Source: CAD feature listing. Evaluate the final solid. Frame: model axes, mm. A direction names the side the tool comes from. Round coordinates to 2 decimals unless told otherwise and drop trailing zeros. Return JSON: item names as keys, results as strings. Group by question number.
```python
from build123d import *
from build123d.topology import SkipClean

# Parameters (mm, degrees)
SKETCH1_R           = 8.984375
SKETCH1_R_2         = 1.984375
SKETCH1_R_3         = 0.75
BOSS_EXTRUDE1_DEPTH = 2
SKETCH6_W           = 17.96875
SKETCH6_H           = 8
CUT_EXTRUDE1_DEPTH  = 16.014592511
BOSS_EXTRUDE3_START = -2
SKETCH7_R           = 1.65
BOSS_EXTRUDE3_DEPTH = 2
SKETCH8_R           = 1.1
BOSS_EXTRUDE4_DEPTH = 1


with BuildPart() as part:
    # Sketch1 → Boss-Extrude1 (new body)
    with BuildSketch(Plane(origin=(0, 0, 0), x_dir=(1, 0, 0), z_dir=(0, 1, 0))):
        with Locations(Location((0, 0, 0), (0, 0, 270))):
            Circle(SKETCH1_R)
        with Locations(Location((0, 0, 0), (0, 0, 270))):
            Circle(SKETCH1_R_2, mode=Mode.SUBTRACT)
        with Locations(Location((0, 7, 0), (0, 0, 270))):
            Circle(SKETCH1_R_3, mode=Mode.SUBTRACT)
        with Locations(Location((5.472820377, 4.364428613, 0), (0, 0, 270))):
            Circle(SKETCH1_R_3, mode=Mode.SUBTRACT)
        with Locations(Location((6.824495385, -1.557646538, 0), (0, 0, 270))):
            Circle(SKETCH1_R_3, mode=Mode.SUBTRACT)
        with Locations(Location((3.037186174, -6.306782075, 0), (0, 0, 270))):
            Circle(SKETCH1_R_3, mode=Mode.SUBTRACT)
        with Locations(Location((-3.037186174, -6.306782075, 0), (0, 0, 270))):
            Circle(SKETCH1_R_3, mode=Mode.SUBTRACT)
        with Locations(Location((-6.824495385, -1.557646538, 0), (0, 0, 270))):
            Circle(SKETCH1_R_3, mode=Mode.SUBTRACT)
        with Locations(Location((-5.472820377, 4.364428613, 0), (0, 0, 270))):
            Circle(SKETCH1_R_3, mode=Mode.SUBTRACT)
    extrude(amount=BOSS_EXTRUDE1_DEPTH)

    # Sweep1: sweep along a path in Sketch3
    with SkipClean():  # the faces are left unmerged after this step: merging them gives an invalid solid
        with BuildLine(Plane(origin=(0, 0, 0), x_dir=(0, 0, -1), z_dir=(1, 0, 0))) as sweep1_path:
            Line((0, 2), (0, 8))
        # Sketch2 → Sweep1 (sweep)
        with BuildSketch(Plane(origin=(0, 2, 0), x_dir=(1, 0, 0), z_dir=(0, 1, 0))):
            with BuildLine():
                Line((-0.5, 6.229967897), (-0.5, 1.920350005))
                ThreePointArc((-0.5, 1.920350005), (-0.860988045, 1.787860097), (-1.18964519, 1.588234385))
                Line((-1.18964519, 1.588234385), (-4.559040136, 4.275237191))
                ThreePointArc((-4.559040136, 4.275237191), (-2.711773369, 5.631055424), (-0.5, 6.229967897))
            make_face()
            with BuildLine():
                Line((0.5, 6.229967897), (0.5, 1.920350005))
                ThreePointArc((0.5, 1.920350005), (0.860988045, 1.787860097), (1.18964519, 1.588234385))
                Line((1.18964519, 1.588234385), (4.559040136, 4.275237191))
                ThreePointArc((4.559040136, 4.275237191), (2.711773369, 5.631055424), (0.5, 6.229967897))
            make_face()
            with BuildLine():
                Line((5.182529938, 3.493405709), (1.813134992, 0.806402903))
                ThreePointArc((1.813134992, 0.806402903), (1.934622576, 0.441564978), (1.983463288, 0.06014588))
                Line((1.983463288, 0.06014588), (6.185030062, -0.898834319))
                ThreePointArc((6.185030062, -0.898834319), (6.093299451, 1.390755837), (5.182529938, 3.493405709))
            make_face()
            with BuildLine():
                Line((5.962509128, -1.873762231), (1.760942354, -0.914782033))
                ThreePointArc((1.760942354, -0.914782033), (1.551446848, -1.237237576), (1.283693074, -1.5132337))
                Line((1.283693074, -1.5132337), (3.1535662, -5.396065254))
                ThreePointArc((3.1535662, -5.396065254), (4.886446765, -3.896811262), (5.962509128, -1.873762231))
            make_face()
            with BuildLine():
                Line((2.252597332, -5.829948993), (0.382724207, -1.947117439))
                ThreePointArc((0.382724207, -1.947117439), (0, -1.984375), (-0.382724207, -1.947117439))
                Line((-0.382724207, -1.947117439), (-2.252597332, -5.829948993))
                ThreePointArc((-2.252597332, -5.829948993), (0, -6.25), (2.252597332, -5.829948993))
            make_face()
            with BuildLine():
                Line((-3.1535662, -5.396065254), (-1.283693074, -1.5132337))
                ThreePointArc((-1.283693074, -1.5132337), (-1.551446848, -1.237237576), (-1.760942354, -0.914782033))
                Line((-1.760942354, -0.914782033), (-5.962509128, -1.873762231))
                ThreePointArc((-5.962509128, -1.873762231), (-4.886446765, -3.896811262), (-3.1535662, -5.396065254))
            make_face()
            with BuildLine():
                Line((-6.185030062, -0.898834319), (-1.983463288, 0.06014588))
                ThreePointArc((-1.983463288, 0.06014588), (-1.934622576, 0.441564978), (-1.813134992, 0.806402903))
                Line((-1.813134992, 0.806402903), (-5.182529938, 3.493405709))
                ThreePointArc((-5.182529938, 3.493405709), (-6.093299451, 1.390755837), (-6.185030062, -0.898834319))
            make_face()
        sweep(path=sweep1_path.line)

    # Sketch4 → Revolve1 (revolve)
    with SkipClean():  # the faces are left unmerged after this step: merging them gives an invalid solid
        with BuildSketch(Plane(origin=(0, 0, 0), x_dir=(0, 0, -1), z_dir=(1, 0, 0)), mode=Mode.PRIVATE) as revolve1_sk:
            Polygon((-5.396065254, 2), (-1.984375, 2), (-1.984375, 8), align=None)
        revolve(revolve1_sk.sketch.rotate(Axis((0, 0, 0), (0, 1, 0)), 165.405971265), axis=Axis((0, 0, 0), (0, 1, 0)))

    # Sketch6 → Cut-Extrude1 (cut, through all)
    with SkipClean():  # the faces are left unmerged after this step: merging them gives an invalid solid
        with BuildSketch(Plane(origin=(0, 0, 0), x_dir=(0.6052939880428899, 0, 0.7960020025346255), z_dir=(-0.7960020025346255, 0, 0.6052939880428899))):
            with Locations((0, 4)):
                Rectangle(SKETCH6_W, SKETCH6_H)
        extrude(amount=-CUT_EXTRUDE1_DEPTH, mode=Mode.SUBTRACT)

    # Sketch7 → Boss-Extrude3 (add)
    with SkipClean():  # the faces are left unmerged after this step: merging them gives an invalid solid
        with BuildSketch(Plane(origin=(0, 2, 0), x_dir=(1, 0, 0), z_dir=(0, 1, 0)).offset(BOSS_EXTRUDE3_START)):
            with BuildLine():
                Line((5.438188174, -7.151580492), (7.839492164, -9.165791707))
                ThreePointArc((7.839492164, -9.165791707), (8.271761308, -14.096627679), (3.340925335, -14.528896823))
                Line((3.340925335, -14.528896823), (-5.773830193, -6.883449647))
                ThreePointArc((-5.773830193, -6.883449647), (-0.214796249, -8.981806985), (5.438188174, -7.151580492))
            make_face()
            with Locations(Location((5.59020875, -11.847344265, 0), (0, 0, 270))):
                Circle(SKETCH7_R, mode=Mode.SUBTRACT)
        extrude(amount=BOSS_EXTRUDE3_DEPTH)

    # Sketch8 → Boss-Extrude4 (add)
    # profile 1 of 2: a face of its own
    with SkipClean():  # the faces are left unmerged after this step: merging them gives an invalid solid
        with BuildSketch(Plane(origin=(0, 0, 0), x_dir=(-0.60529398804289, 0, -0.7960020025346255), z_dir=(0.7960020025346254, 0, -0.6052939880428899))):
            with BuildLine():
                ThreePointArc((-8.25, 6.5), (-10.017766953, 5.767766953), (-10.75, 4))
                Line((-10.75, 4), (-10.75, 2))
                Line((-10.75, 2), (-5.75, 2))
                Line((-5.75, 2), (-5.75, 6.5))
                Line((-5.75, 6.5), (-8.25, 6.5))
            make_face()
            with Locations((-8.25, 4)):
                Circle(SKETCH8_R, mode=Mode.SUBTRACT)
        # profile 2 of 2: a face of its own
        with BuildSketch(Plane(origin=(0, 0, 0), x_dir=(-0.60529398804289, 0, -0.7960020025346255), z_dir=(0.7960020025346254, 0, -0.6052939880428899))):
            with BuildLine():
                Line((5.75, 2), (8.484375, 2))
                Line((8.484375, 2), (8.484375, 0))
                Line((8.484375, 0), (10.75, 0))
                Line((10.75, 0), (10.75, 4))
                ThreePointArc((10.75, 4), (10.017766953, 5.767766953), (8.25, 6.5))
                Line((8.25, 6.5), (5.75, 6.5))
                Line((5.75, 6.5), (5.75, 2))
            make_face()
            with Locations((8.25, 4)):
                Circle(SKETCH8_R, mode=Mode.SUBTRACT)
        extrude(amount=-BOSS_EXTRUDE4_DEPTH)


solid = part.part
```
(1) Mould query, pull axis X, two halves, no side actions, for faces 1 (the face through (-4.299, 5.709, 1.494)), 2 (the face through (8.32, 0.99, 14.04)), 3 (the face through (-2.61, 5.62, -2.08)). Classes: released by +X, released by -X, zero draft, split by the parting line, or undercut.
(2) Set-up query: faces 4 (the face through (-8.983, 0.986, 0.18)), 5 (the face through (-6.086, 5.042, -1.422)), 6 (the face through (-2.44, 5.71, 3.91)), 7 (the face through (3.5, 2, 6)). Return all of +Z, -Z, +X, -X, +Y, -Y with unobstructed straight access to the full face (end or side cutting, diameter ignored); none if empty.
(3) Pin query (flat end, axial travel): pin 1 (1.4 mm diameter, centred on x = 3.04, z = 6.31, fed in from +Y); pin 2 (2.5 mm diameter, centred on x = -0.5, z = 11, fed in from +Y); pin 3 (3.5 mm diameter, centred on x = 0, z = 0, fed in from +Y). Return the tip coordinate at first contact, or that it passes through.
(4) Ray query, line 1 (Z direction, x = -2.75, y = 7.5); line 2 (Y direction, x = -7.25, z = 5); line 3 (Z direction, x = 1.5, y = 6.5). Return the intervals inside material, ascending.
Answers follow:
{
 "1": {"face 1": "released by -X", "face 2": "split by the parting line", "face 3": "undercut"},
 "2": {"face 4": "-X, +Y, -Y", "face 5": "-X, +Y", "face 6": "+Y", "face 7": "-Y"},
 "3": {"pin 1": "y = 6.5", "pin 2": "y = 2", "pin 3": "through"},
 "4": {"line 1": "-3.62 to -2.83, -1.55 to 0.11, 1.14 to 4.56", "line 2": "0 to 2", "line 3": "1.97 to 2.41, 4.27 to 6.07"}
}
